Geometry check sheet. Reference: drawing and pictorial views, mm from the part's lowest x, y, z. Coordinates: 2 decimals unless noted, no trailing zeros. Loops run counter-clockwise (first coordinate to the right, second up) from the corner with the lowest first, then second, coordinate; pieces in that order, holes last. Notation, with made-up numbers: (-28.75, 79) -> (12.25, 79) arc R33 cw to (12.25, 113) -> close; hole circle Ø11 at (-26, 35.25). An arc over 180 degrees is marked (long way). Use one line per item in the form item = value.
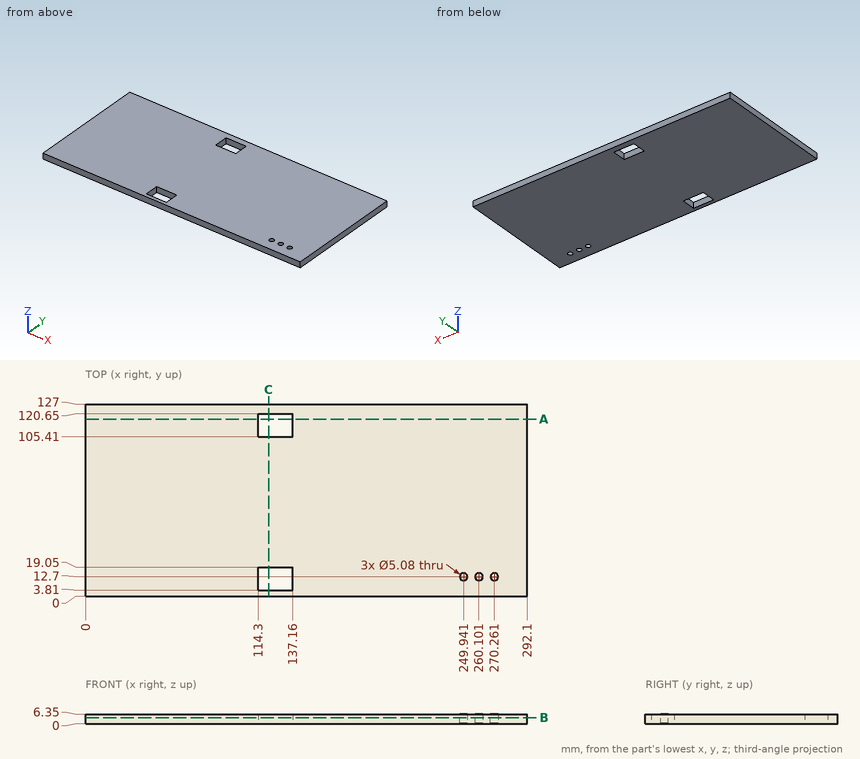
(1) Section check B-B, the plane z = 4. Record the boundary of the cut face in (x, y).
Established:
outline = (0, 0) -> (292.1, 0) -> (292.1, 127) -> (0, 127) -> close; hole (114.3, 3.81) -> (137.16, 3.81) -> (137.16, 19.05) -> (114.3, 19.05) -> close; hole (114.3, 105.41) -> (137.16, 105.41) -> (137.16, 120.65) -> (114.3, 120.65) -> close; hole circle Ø5.08 at (249.94, 12.7); hole circle Ø5.08 at (260.1, 12.7); hole circle Ø5.08 at (270.26, 12.7)
(2) Scan lines: line 1 along Y through (x, z) = (128, 3.25); line 2 along X through (y, z) = (19, 6); line 3 along X through (y, z) = (14, 2.5). Record each from-to range of solid material in increasing order.
Established:
line_1 = 0 to 3.81, 19.05 to 105.41, 120.65 to 127
line_2 = 0 to 114.3, 137.16 to 292.1
line_3 = 0 to 114.3, 137.16 to 247.76, 252.12 to 257.92, 262.28 to 268.08, 272.44 to 292.1
(3) Section check C-C, the plane x = 121. Record the boundary of the cut face in (y, z), plus the area to 3 significant figures.
Established:
outline = (0, 0) -> (3.81, 0) -> (3.81, 6.35) -> (0, 6.35) -> close; (19.05, 0) -> (105.41, 0) -> (105.41, 6.35) -> (19.05, 6.35) -> close; (120.65, 0) -> (127, 0) -> (127, 6.35) -> (120.65, 6.35) -> close
area = 613 mm²
(4) Section check A-A, the plane y = 117. Record the boundary of the cut face in (x, z).
Established:
outline = (0, 0) -> (114.3, 0) -> (114.3, 6.35) -> (0, 6.35) -> close; (137.16, 0) -> (292.1, 0) -> (292.1, 6.35) -> (137.16, 6.35) -> close
